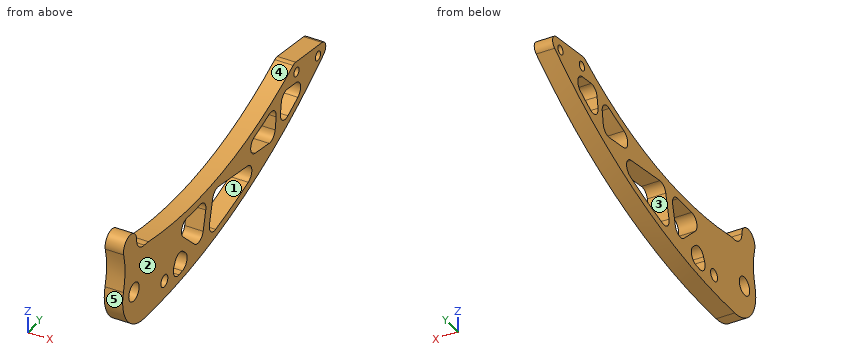
from build123d import *

# Parameters (mm, degrees)
SKETCH1_R           = 6
BOSS_EXTRUDE1_DEPTH = 12
SKETCH3_R           = 3
CUT_EXTRUDE2_DEPTH  = 13
CUT_EXTRUDE3_DEPTH  = 13
FILLET1_R           = 6
SKETCH2_R           = 4
CUT_EXTRUDE1_DEPTH  = 13.0000001
SKETCH5_R           = 7.5
BOSS_EXTRUDE2_DEPTH = 12
FILLET2_R           = 5


with BuildPart() as part:
    # Sketch1 → Boss-Extrude1 (new body)
    with BuildSketch(Plane(origin=(0, 0, 0), x_dir=(0, 0, -1), z_dir=(1, 0, 0))):
        with BuildLine():
            ThreePointArc((24.992781164, -0.60074095), (9.243822678, 113.703988064), (-41.858816097, 217.155044504))
            Line((-41.858816097, 217.155044504), (-48.12160564, 172.59298141))
            ThreePointArc((-48.12160564, 172.59298141), (-22.274376436, 90.661190514), (-24.538993202, 4.778892408))
            ThreePointArc((-24.538993202, 4.778892408), (2.400538477, 24.88448141), (25, 0))
            ThreePointArc((25, 0), (24.998195226, -0.30039216), (24.992781164, -0.60074095))
        make_face()
        with BuildLine():
            ThreePointArc((-24.538993202, 4.778892408), (-2.699369305, -24.853840857), (24.992781164, -0.60074095))
            ThreePointArc((24.992781164, -0.60074095), (24.998195226, -0.30039216), (25, 0))
            ThreePointArc((25, 0), (2.400538477, 24.88448141), (-24.538993202, 4.778892408))
        make_face()
        with Locations((0, -12)):
            Circle(SKETCH1_R, mode=Mode.SUBTRACT)
    extrude(amount=BOSS_EXTRUDE1_DEPTH)

    # Sketch3 → Cut-Extrude2 (cut, through all)
    with BuildSketch(Plane(origin=(12, 0, 0), x_dir=(0, 0, -1), z_dir=(1, 0, 0))):
        with Locations((-40.714528231, 175)):
            Circle(SKETCH3_R)
        with Locations((-37.235200707, 199.756701719)):
            Circle(SKETCH3_R)
    extrude(amount=-CUT_EXTRUDE2_DEPTH, mode=Mode.SUBTRACT)

    # Sketch4 → Cut-Extrude3 (cut, through all)
    with BuildSketch(Plane(origin=(12, 0, 0), x_dir=(0, 0, -1), z_dir=(1, 0, 0))):
        with BuildLine():
            ThreePointArc((-11.749836025, 155.008629259), (-20.960958666, 173.77628952), (-31.260870979, 191.969190837))
            Line((-31.260870979, 191.969190837), (-35.976814508, 158.413509038))
            Line((-35.976814508, 158.413509038), (-11.749836025, 155.008629259))
        make_face()
        with BuildLine():
            Line((-9.354323007, 149.622823998), (-33.760235475, 153.052851308))
            ThreePointArc((-33.760235475, 153.052851308), (-24.416431689, 125.419954523), (-18.166319592, 96.927503721))
            Line((-18.166319592, 96.927503721), (-9.354323007, 149.622823998))
        make_face()
        with BuildLine():
            ThreePointArc((14.161868129, 72.691486719), (5.930300275, 107.334766496), (-5.730334656, 140.979158838))
            Line((-5.730334656, 140.979158838), (-15.958464631, 79.815428272))
            Line((-15.958464631, 79.815428272), (14.161868129, 72.691486719))
        make_face()
        with BuildLine():
            Line((15.468075791, 65.189422352), (-15.356589243, 72.479949778))
            ThreePointArc((-15.356589243, 72.479949778), (-14.750380465, 52.717361117), (-15.619336812, 32.964581198))
            Line((-15.619336812, 32.964581198), (15.468075791, 65.189422352))
        make_face()
        with BuildLine():
            ThreePointArc((19.721068997, 24.377203305), (18.614609922, 40.455333735), (16.779570125, 56.466678425))
            Line((16.779570125, 56.466678425), (-2, 37))
            ThreePointArc((-2, 37), (10.561248293, 33.615157675), (19.721068997, 24.377203305))
        make_face()
    extrude(amount=-CUT_EXTRUDE3_DEPTH, mode=Mode.SUBTRACT)

    # Fillet1
    fillet1_edges = [part.edges().sort_by_distance(p)[0] for p in [
        (6, 155.008629259, 11.749836025),
        (6, 158.413509038, 35.976814508),
        (6, 191.969190837, 31.260870979),
        (6, 96.927503721, 18.166319592),
        (6, 153.052851308, 33.760235475),
        (6, 149.622823998, 9.354323007),
        (6, 72.691486719, -14.161868129),
        (6, 79.815428272, 15.958464631),
        (6, 140.979158838, 5.730334656),
        (6, 32.964581198, 15.619336812),
        (6, 72.479949778, 15.356589243),
        (6, 65.189422352, -15.468075791),
        (6, 24.377203305, -19.721068997),
        (6, 37, 2),
        (6, 56.466678425, -16.779570125),
    ]]
    fillet(fillet1_edges, radius=FILLET1_R)

    # Sketch2 → Cut-Extrude1 (cut, through all)
    with BuildSketch(Plane(origin=(12, 0, 0), x_dir=(0, 0, -1), z_dir=(1, 0, 0))):
        with Locations((13, 23)):
            Circle(SKETCH2_R)
    extrude(amount=-CUT_EXTRUDE1_DEPTH, mode=Mode.SUBTRACT)

    # Sketch5 → Boss-Extrude2 (add)
    with BuildSketch(Plane(origin=(12, 0, 0), x_dir=(0, 0, -1), z_dir=(1, 0, 0))):
        with BuildLine():
            ThreePointArc((-34, -9), (-28.696699141, -11.196699141), (-26.5, -16.5))
            ThreePointArc((-26.5, -16.5), (-28.087357429, -21.114180081), (-32.177508753, -23.775199355))
            ThreePointArc((-32.177508753, -23.775199355), (-19.40613231, -22.280390349), (-6.675855702, -24.092176129))
            ThreePointArc((-6.675855702, -24.092176129), (-19.898447082, -15.134457497), (-25, 0))
            ThreePointArc((-25, 0), (-27.636038969, -6.363961031), (-34, -9))
        make_face()
        with Locations((-34, -16.5)):
            Circle(SKETCH5_R)
    extrude(amount=-BOSS_EXTRUDE2_DEPTH)

    # Fillet2
    fillet2_edges = [part.edges().sort_by_distance(p)[0] for p in [
        (6, 172.59298141, 48.12160564),
        (6, 217.155044504, 41.858816097),
    ]]
    fillet(fillet2_edges, radius=FILLET2_R)


solid = part.part
Build history of the part. All positions in model axes, mm. Face numbers are marked on the shaded views. A direction names the side the tool comes from. Give positions to 0.01 mm unless a question says otherwise; leave off trailing zeros. Order: outer loops, then holes, each group sorted by start corner. A loop starts at its lowest first (then second) coordinate and runs counter-clockwise, first axis right, second up. Notation, with made-up numbers: M 39,17.5 L 85,17.5 A21 cw 85,30.5 Z; hole C 53,67.5 d11. An arc over 180 degrees is marked long. Use one line per item in the form item = value.
1) Saw through at B-B (z = 0). Give the cut face in (x, y).
Calculated:
outline = M 0,-25 L 12,-25 L 12,-18 L 0,-18 Z; M 0,-6 L 12,-6 L 12,49.16 L 0,49.16 Z; M 0,68.85 L 12,68.85 L 12,76.04 L 0,76.04 Z; M 0,122.46 L 12,122.46 L 12,140.11 L 0,140.11 Z
2) Tool access for the marked faces 1 and 2: list every direction of +Z, -Z, +X, -X, +Y, -Y with a clear straight run to the whole face (end or side of a thin tool).
Calculated:
face_1 = +X, -X
face_2 = +Z, -Z, +X, +Y, -Y
3) Saw through at A-A (y = 23). Give the cut face in (x, z), plus the area to 3 significant figures.
Calculated:
outline = M 0,-24.79 L 12,-24.79 L 12,-17 L 0,-17 Z; M 0,-9 L 12,-9 L 12,21.66 L 0,21.66 Z
area = 461 mm2
4) Drop flat-ended pins along their axis: pin 1 (5 mm diameter, centred on x = 7, z = 31.5, fed in from +Y); pin 2 (3 mm diameter, centred on x = 4, y = 5, fed in from -Z); pin 3 (5 mm diameter, centred on x = 10, z = 26.5, fed in from +Y). Give the stop position or say it passes through.
Calculated:
pin_1 = 205.68
pin_2 = -25.09
pin_3 = 197.85
5) Probe probe 1 along Y at (x, z) = (6, 19); probe 2 along Y at (x, z) = (2.25, 17); probe 3 along Z at (x, y) = (10.25, 46). List the from-to ranges inside material, lowest first.
Calculated:
probe_1 = -22.29 to 122.32, 150.98 to 157.27, 170.01 to 180.69
probe_2 = -22.37 to 122.67, 150.7 to 159.09, 166.05 to 176.98
probe_3 = -23.09 to -17.63, -6.68 to 3.04, 14.18 to 19.88
6) Two-plate mould, pull along Z, no slides. Class the marked faces 3, 4 and 5: released by +Z, released by -Z, zero draft, split by the parting line, or undercut.
Calculated:
face_3 = undercut
face_4 = released by +Z
face_5 = split by the parting line
7) Saw through at D-D (x = 7.75). State how many separate pieces and enclosed holes the cut face has, plus the area to 3 significant figures.
Calculated:
separate_pieces = 1
enclosed_holes = 9
area = 6,250 mm2
8) Saw through at C-C (y = -12). Give the cut face in (x, z), plus the area to 3 significant figures.
Calculated:
outline = M 0,-21.93 L 12,-21.93 L 12,-6 L 0,-6 Z; M 0,6 L 12,6 L 12,40 L 0,40 Z
area = 599 mm2
